from build123d import *

# Parameters (mm, degrees)
SKETCH_1_W          = 77
SKETCH_1_H          = 45
EXTRUDE_1_DEPTH     = 33
CUT_EXTRUDE_1_DEPTH = 30
SKETCH_5_W          = 18
SKETCH_5_H          = 3
EXTRUDE_3_DEPTH     = 20
EXTRUDE_4_DEPTH     = 3
SKETCH_8_W          = 41
SKETCH_8_H          = 3
EXTRUDE_6_DEPTH     = 10
SKETCH_4_R          = 3.25
EXTRUDE_2_DEPTH     = 15


with BuildPart() as part:
    # 草图1 → 凸台-拉伸1 (new body)
    with BuildSketch(Plane(origin=(0, 0, 0), x_dir=(1, 0, 0), z_dir=(0, 1, 0))):
        Rectangle(SKETCH_1_W, SKETCH_1_H)
    extrude(amount=EXTRUDE_1_DEPTH)

    # 草图2 → 切除-拉伸1 (cut)
    with BuildSketch(Plane(origin=(0, 33, 0), x_dir=(1, 0, 0), z_dir=(0, 1, 0))):
        Polygon((35.5, -19.5), (35.5, 19.5), (-35.5, 19.5), (-35.5, -19.5), (-20.5, -19.5), (-20.5, -22.5), (20.5, -22.5), (20.5, -19.5), align=None)
    extrude(amount=-CUT_EXTRUDE_1_DEPTH, mode=Mode.SUBTRACT)

    # 草图5 → 凸台-拉伸3 (add)
    with BuildSketch(Plane(origin=(0, 33, 0), x_dir=(1, 0, 0), z_dir=(0, 1, 0))):
        with Locations((-29.5, -21)):
            Rectangle(SKETCH_5_W, SKETCH_5_H)
        with Locations((29.5, -21)):
            Rectangle(SKETCH_5_W, SKETCH_5_H)
    extrude(amount=EXTRUDE_3_DEPTH)

    # 草图7 → 凸台-拉伸4 (add)
    with BuildSketch(Plane(origin=(38.5, 0, 0), x_dir=(0, 0, -1), z_dir=(1, 0, 0))):
        Polygon((22.5, 33), (-19.5, 33), (-19.5, 53), align=None)
    extrude_4 = extrude(amount=-EXTRUDE_4_DEPTH)

    # 镜向1: 凸台-拉伸4 across plane
    add(extrude_4.mirror(Plane(origin=(0, 0, 0), x_dir=(0, 0, 1), z_dir=(1, 0, 0))))

    # 草图8 → 凸台-拉伸6 (add)
    with BuildSketch(Plane(origin=(0, 3, 0), x_dir=(1, 0, 0), z_dir=(0, 1, 0))):
        with Locations((0, -21)):
            Rectangle(SKETCH_8_W, SKETCH_8_H)
    extrude(amount=EXTRUDE_6_DEPTH)

    # 草图4 → 凸台-拉伸2 (add)
    # profile 1 of 2: a face of its own
    with BuildSketch(Plane(origin=(0, 0, 0), x_dir=(1, 0, 0), z_dir=(0, 1, 0))):
        with BuildLine():
            Line((-37.5, -27.5), (-37.5, -22.5))
            Line((-37.5, -22.5), (-24.5, -22.5))
            Line((-24.5, -22.5), (-24.5, -27.5))
            ThreePointArc((-24.5, -27.5), (-31, -34), (-37.5, -27.5))
        make_face()
        with Locations(Location((-31, -27.5, 0), (0, 0, 270))):
            Circle(SKETCH_4_R, mode=Mode.SUBTRACT)
    # profile 2 of 2: a face of its own
    with BuildSketch(Plane(origin=(0, 0, 0), x_dir=(1, 0, 0), z_dir=(0, 1, 0))):
        with BuildLine():
            Line((37.5, -27.5), (37.5, -22.5))
            Line((37.5, -22.5), (24.5, -22.5))
            Line((24.5, -22.5), (24.5, -27.5))
            ThreePointArc((24.5, -27.5), (31, -34), (37.5, -27.5))
        make_face()
        with Locations(Location((31, -27.5, 0), (0, 0, 270))):
            Circle(SKETCH_4_R, mode=Mode.SUBTRACT)
    extrude(amount=EXTRUDE_2_DEPTH)


solid = part.part
Model file for the job. Use its own axes, mm. A direction names the side the tool comes from. Give positions to 0.01 mm unless a question says otherwise; leave off trailing zeros. Order: outer loops, then holes, each group sorted by start corner. A loop starts at its lowest first (then second) coordinate and runs counter-clockwise, first axis right, second up. Notation, with made-up numbers: (-18, 65) - (28, 65) arc R18 ccw to (28, 85) - close; hole circle Ø1 at (79.25, 56). An arc over 180 degrees is marked (long way). Return JSON: item names as keys, results as strings.
1) Cut at D-D, the plane y = 34. Give the cut face in (x, z), plus the area to 3 significant figures.
Geometry says:
{"outline": "(-38.5, -20.4) - (-35.5, -20.4) - (-35.5, 19.5) - (-20.5, 19.5) - (-20.5, 22.5) - (-38.5, 22.5) - close; (20.5, 19.5) - (35.5, 19.5) - (35.5, -20.4) - (38.5, -20.4) - (38.5, 22.5) - (20.5, 22.5) - close", "area": "347 mm²"}
2) 3-axis set-ups, long thin cutter, end or side, ignore diameter. For faces 1 (the flat face through (-24.5, 7, 25)), 2 (the flat face through (-20.5, 33, 21)), 3 (the flat face through (0, 3, 0)), 4 (the flat face through (33.8, 15, 29.45)): which of +Z, -Z, +X, -X, +Y, -Y reach the whole face in a straight line?
Geometry says:
{"face 1": "+Z, +Y, -Y", "face 2": "+Z, +Y", "face 3": "+Y", "face 4": "+Z, +X, -X, +Y"}
3) Cut at B-B, the plane x = -31. Give the cut face in (y, z), plus the area to 3 significant figures.
Geometry says:
{"outline": "(0, -22.5) - (33, -22.5) - (33, -19.5) - (3, -19.5) - (3, 19.5) - (53, 19.5) - (53, 22.5) - (15, 22.5) - (15, 24.25) - (0, 24.25) - close; (0, 30.75) - (15, 30.75) - (15, 34) - (0, 34) - close", "area": "450 mm²"}
4) Probe line 1 (Z direction, x = -29, y = 27); line 2 (X direction, y = 14, z = 1); line 3 (X direction, y = 28, z = 21.5). List the from-to ranges inside material, lowest first. Write a range as from..to.
Geometry says:
{"line 1": "-22.5..-19.5, 19.5..22.5", "line 2": "-38.5..-35.5, 35.5..38.5", "line 3": "-38.5..-20.5, 20.5..38.5"}
5) Pull direction X, two halves, no side cores. Call faces 5 (the flat face through (0, 18, -19.5)), 6 (the flat face through (29, 53, 21)), 7 (the flat face through (-38.5, 21, 0)), 8 (the flat face through (37.5, 7, 25)): pulls with the +X half, pulls with the -X half, needs draft (parallel to the pull), parting line crosses it, or undercut.
Geometry says:
{"face 5": "undercut", "face 6": "needs draft", "face 7": "pulls with the -X half", "face 8": "pulls with the +X half"}
6) Cut at C-C, the plane z = 29. Give the cut face in (x, y).
Geometry says:
{"outline": "(-37.32, 0) - (-33.88, 0) - (-33.88, 15) - (-37.32, 15) - close; (-28.12, 0) - (-24.68, 0) - (-24.68, 15) - (-28.12, 15) - close; (24.68, 0) - (28.12, 0) - (28.12, 15) - (24.68, 15) - close; (33.88, 0) - (37.32, 0) - (37.32, 15) - (33.88, 15) - close"}
7) Flat gauge pins, fed straight in: P1, Ø1, axis at x = -28, y = 24.5, coming from the +Z side; P2, Ø1.5, axis at y = 8.5, z = 24.5, coming from the -X side; P3, Ø0.9, axis at x = -11.5, z = -20.5, coming from the +Y side; P4, Ø10, axis at y = 27, z = 24.5, coming from the +X side. Where does each tip first touch, or does it go through?
Geometry says:
{"P1": "z = 22.5", "P2": "x = -37.5", "P3": "y = 33", "P4": "x = 38.5"}
8) Cut at A-A, the plane y = 43. Give the cut face in (x, z).
Geometry says:
{"outline": "(-38.5, -1.5) - (-35.5, -1.5) - (-35.5, 19.5) - (-20.5, 19.5) - (-20.5, 22.5) - (-38.5, 22.5) - close; (20.5, 19.5) - (35.5, 19.5) - (35.5, -1.5) - (38.5, -1.5) - (38.5, 22.5) - (20.5, 22.5) - close"}
